Autodesk Inventor part; units mm, degrees
ref_plane "YZ Plane" through (0, 0, 0) normal (1, 0, 0) x (0, 1, 0)
ref_plane "XZ Plane" through (0, 0, 0) normal (0, 1, 0) x (-1, 0, 0)
ref_plane "XY Plane" through (0, 0, 0) normal (0, 0, 1) x (1, 0, 0)
sketch "Sketch1" plane through (0, 0, 0) normal (0, 1, 0) x (-1, 0, 0)
  circle A0 centre (0, 0) radius 4.1275
  dimension "d0" = 8.255
extrude "Extrusion1" add sketch "Sketch1" along normal blind 10.795
shell "Shell1" thickness 0.635 removed faces 1 at (0.4879, 0, 1.9449)
fillet "Fillet1" radius 1.5875 1 edges at (4.1275, 10.795, 0)
properties part number "buttom piston" material "PBT Plastic"
Work out the finished part from the listing and answer in its coordinate system (mm). Round coordinates to 2 decimals unless told otherwise and drop trailing zeros. Write each loop counter-clockwise with the first axis right and the second up, starting at its lowest first coordinate (ties: lowest second). Pieces come first, ordered by that corner, then holes. Notation, with made-up numbers: (-16, 47) -> (26, 47) arc R15 ccw to (26, 63) -> close; hole circle Ø3 at (-11.75, 76). An arc over 180 degrees is marked (long way). Write each question's results on one line, items separated by ' | '.
Item 1: A cutting plane is placed at A-A, the plane z = 0. Determine the outline of the cut face in (x, y) (1 decimal), plus the area to 3 significant figures.
Result set:
outline: (-4.1, 0) -> (-3.5, 0) -> (-3.5, 10.2) -> (3.5, 10.2) -> (3.5, 0) -> (4.1, 0) -> (4.1, 9.2) arc R1.6 ccw to (2.5, 10.8) -> (-2.5, 10.8) arc R1.6 ccw to (-4.1, 9.2) -> close | area: 17.1 mm^2
Item 2: The mould has two halves that part along X. Classify faces 1 (the face through (0, 10.795, 0)), 2 (the face through (0, 10.16, 0)), 3 (the face through (0.455, 5.009, -3.463)), 4 (the face through (-3.937, 4.539, -1.24)): +X half, -X half, draft (parallel to the pull), parting line (faces both ways), or undercut.
Result set:
face 1: draft | face 2: undercut | face 3: undercut | face 4: parting line
Item 3: Find the intervals of material crossed by line 1 along Z through (x, y) = (0, 6); line 2 along Y through (x, z) = (1.5, -1.25) (3 decimals); line 3 along Z through (x, y) = (1, 3), in increasing order. Write a range as [from, to].
Result set:
line 1: [-4.13, -3.49], [3.49, 4.13] | line 2: [10.16, 10.795] | line 3: [-4, -3.35], [3.35, 4]
Item 4: Flat-ended cylindrical pins translate along their axes: P1, Ø1.5, axis at x = -1.5, y = 5, coming from the +Z side; P2, Ø1.5, axis at x = 3, y = 5, coming from the -Z side. Find the tip coordinate at first contact, or state that the pin passes through.
Result set:
P1: z = 4.06 | P2: z = -3.46
Item 5: A cutting plane is placed at B-B, the plane y = 6.75. Determine the outline of the cut face in (x, z) (1 decimal).
Result set:
outline: circle Ø8.3 at (0, 0); hole circle Ø7 at (0, 0)
Item 6: A cutting plane is placed at C-C, the plane y = 9.5. Determine the outline of the cut face in (x, z) (1 decimal), plus the area to 3 significant figures.
Result set:
outline: circle Ø8.2 at (0, 0); hole circle Ø7 at (0, 0) | area: 14.5 mm^2
